The model under review builds one solid part; all positions refer to its coordinate system, in mm. A direction names the side the tool comes from. Give positions to 0.01 mm unless a question says otherwise; leave off trailing zeros. Loops run counter-clockwise (first coordinate to the right, second up) from the corner with the lowest first, then second, coordinate; pieces in that order, holes last. Notation, with made-up numbers: M 43.5,-38 L 83.5,-38 A28 cw 83.5,-15 Z; hole C 29,-30 d8. An arc over 180 degrees is marked long. Return JSON: item names as keys, results as strings.
```python
from build123d import *

# Parameters (mm, degrees)
F1_DEPTH = 30
F3_DEPTH = 10
F5_DEPTH = 40


with BuildPart() as f1:
    # F0 (on Front) → F1 (new body)
    with BuildSketch(Plane.XZ):
        Polygon((-31.843803, -24.386245), (-43.517503, -36.059944), (36.482497, -36.059944), (22.543686, -22.121133), (12.543686, -22.121133), (12.543686, 5.613755), (-21.843803, 5.613755), (-21.843803, -24.386245), align=None)
    extrude(amount=F1_DEPTH)

    # F2 (on face) → F3 (join)
    with BuildSketch(Plane.XZ.offset(30)):
        with BuildLine():
            Line((12.543686, 5.613755), (-21.843803, 5.613755))
            ThreePointArc((-21.843803, 5.613755), (-4.650059, -11.579989), (12.543686, 5.613755))
        make_face()
    extrude(amount=F3_DEPTH)

    # F4 (on face) → F5 (cut)
    with BuildSketch(Plane.XZ.offset(40)):
        with BuildLine():
            Line((-4.650059, 5.613755), (-13.246931, 5.613755))
            ThreePointArc((-13.246931, 5.613755), (-4.650059, -3.024393), (3.946813, 5.613755))
            Line((3.946813, 5.613755), (-4.650059, 5.613755))
        make_face()
    extrude(amount=-F5_DEPTH, mode=Mode.SUBTRACT)


solid = f1.part
```
1) Consider section A-A on z = 2.5. Write out the cut boundary in (x, y).
From the geometry:
{"outline": "M -21.84,-30 L -21.56,-30 L -21.56,-40 L -12.68,-40 L -12.68,0 L -21.84,0 Z; M 3.38,-40 L 12.26,-40 L 12.26,-30 L 12.54,-30 L 12.54,0 L 3.38,0 Z"}
2) Consider section C-C on x = -26. Write out the cut boundary in (y, z).
From the geometry:
{"outline": "M -30,-36.06 L 0,-36.06 L 0,-24.39 L -30,-24.39 Z"}
3) Consider section B-B on y = -20.5. Write out the cut boundary in (x, z).
From the geometry:
{"outline": "M -43.52,-36.06 L 36.48,-36.06 L 22.54,-22.12 L 12.54,-22.12 L 12.54,5.61 L 3.95,5.61 A8.6 cw long -13.25,5.61 L -21.84,5.61 L -21.84,-24.39 L -31.84,-24.39 Z"}
4) Tool access review of faces 1 (the face through (-5.028, -34.93, -11.576)), 2 (the face through (18, -15, -22.121)), 3 (the face through (-27, -15, -24.386)), 4 (the face through (-17, -20, 5.614)), 5 (the face through (-4, 0, -20)): name each direction out of +Z, -Z, +X, -X, +Y, -Y from which nothing blocks a thin tool from reaching the whole face with its end or side.
From the geometry:
{"face 1": "-Z, -Y", "face 2": "+Z, +X, +Y, -Y", "face 3": "+Z, -X, +Y, -Y", "face 4": "+Z, +X, -X, +Y, -Y", "face 5": "+Z, -Z, +X, -X, +Y"}
5) Insertion check: pin 1 (10 mm diameter, centred on y = -20, z = -29.5, fed in from -X); pin 2 (3 mm diameter, centred on y = -31, z = -31.5, fed in from -X); pin 3 (4 mm diameter, centred on x = 18.5, z = -21.5, fed in from -Y). Each pin has a flat end and moves straight along its axis. Give the tip position at first contact, or say it passes through.
From the geometry:
{"pin 1": "x = -41.96", "pin 2": "x = -40.08", "pin 3": "y = -30"}
6) Wall thickness on L1, parallel to X at y = -12.5, z = 4.5; L2, parallel to Y at x = 15, z = -26.5; L3, parallel to X at y = -32, z = 4: over which ranges is each line inside the solid? List them lowest first. Write a range as from..to.
From the geometry:
{"L1": "-21.84..-13.18, 3.88..12.54", "L2": "-30..0", "L3": "-21.77..-13.1, 3.8..12.47"}
7) Consider section D-D on z = -10.5. Write out the cut boundary in (x, y), then the cut area to 3 significant figures.
From the geometry:
{"outline": "M -21.84,-30 L -10.65,-30 L -10.65,-40 L 1.35,-40 L 1.35,-30 L 12.54,-30 L 12.54,0 L -21.84,0 Z", "area": "1,150 mm²"}
8) The part is to be moulded in two halves that separate along X. For faces 6 (the face through (-21.844, -15, -9)), 7 (the face through (-4.84, -20.28, -3.022)), 8 (the face through (-5, -40, -5)), say which applies: released by +X, released by -X, zero draft, split by the parting line, or undercut.
From the geometry:
{"face 6": "released by -X", "face 7": "undercut", "face 8": "zero draft"}
